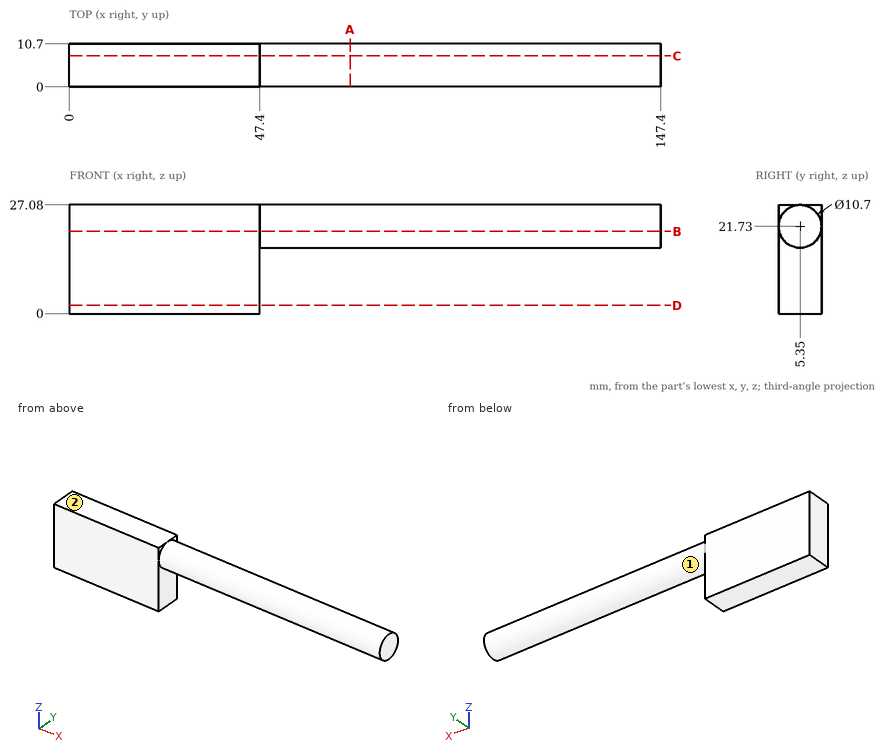
Could you check a few things on this drawing? It's one solid part, dimensions in mm from its lowest x, y, z. A direction names the side the tool comes from. Give positions to 0.01 mm unless a question says otherwise; leave off trailing zeros. Order: outer loops, then holes, each group sorted by start corner. A loop starts at its lowest first (then second) coordinate and runs counter-clockwise, first axis right, second up. Notation, with made-up numbers: (-5.5, 88.5) -> (35.5, 88.5) arc R22 ccw to (35.5, 119.5) -> close; hole circle Ø1 at (34.5, 20.5). An arc over 180 degrees is marked (long way). Answer in a Markdown table with one row per item. Add a question column.
Item 1: Imagine slicing it at D-D (z = 2). List the corners of the cut face in (x, y) for me.
Item 2: Imagine slicing it at C-C (y = 7.75). List the corners of the cut face in (x, z) for me, and give its area (3 significant figures).
Item 3: I'm going to push flat-ended pins straight in: P1, Ø6, axis at x = 122.5, y = 3.5, coming from the -Z side; P2, Ø5.5, axis at y = 4.5, z = 11, coming from the +X side; P3, Ø1, axis at x = 126, z = 14.5, coming from the +Y side. Where does each tip first touch, or does it pass through?
Item 4: Imagine slicing it at B-B (z = 20.5). List the corners of the cut face in (x, y) for me, and give its area (3 significant figures).
Item 5: Imagine slicing it at A-A (x = 70). List the corners of the cut face in (y, z) for me.
Item 6: Please list where these lines run through material, in increasing order: probe 1 along X at (y, z) = (2, 14.75); probe 2 along Z at (x, y) = (112, 5.75); probe 3 along Z at (x, y) = (76, 4).
Item 7: For the marked faces 1 and 2, which set-ups out of +Z, -Z, +X, -X, +Y, -Y let a thin tool reach every point of the face, with its end or its side?
Result:
| question | item | result |
|---|---|---|
| 1 | outline | (0, 0) -> (47.4, 0) -> (47.4, 10.7) -> (0, 10.7) -> close |
| 2 | outline | (0, 0) -> (47.4, 0) -> (47.4, 16.95) -> (147.4, 16.95) -> (147.4, 26.51) -> (47.4, 26.51) -> (47.4, 27.08) -> (0, 27.08) -> close |
| 2 | area | 2,240 mm2 |
| 3 | P1 | z = 16.38 |
| 3 | P2 | x = 47.4 |
| 3 | P3 | through |
| 4 | outline | (0, 0) -> (47.4, 0) -> (47.4, 0.14) -> (147.4, 0.14) -> (147.4, 10.56) -> (47.4, 10.56) -> (47.4, 10.7) -> (0, 10.7) -> close |
| 4 | area | 1,550 mm2 |
| 5 | outline | circle Ø10.7 at (5.35, 21.73) |
| 6 | probe 1 | 0 to 47.4 |
| 6 | probe 2 | 16.39 to 27.07 |
| 6 | probe 3 | 16.55 to 26.91 |
| 7 | face 1 | +X |
| 7 | face 2 | +Z, +X, -X, +Y, -Y |
